Can you work these out from the drawing? Everything is in mm from the part's minimum corner. A direction names the side the tool comes from. Round coordinates to 2 decimals unless told otherwise and drop trailing zeros. Loops run counter-clockwise (first coordinate to the right, second up) from the corner with the lowest first, then second, coordinate; pieces in that order, holes last. Notation, with made-up numbers: (-3, 16) - (38, 16) arc R24 cw to (38, 31) - close; hole circle Ø4 at (56.5, 42.25). An arc over 180 degrees is marked (long way). Return JSON: item names as keys, results as strings. Group by question number.
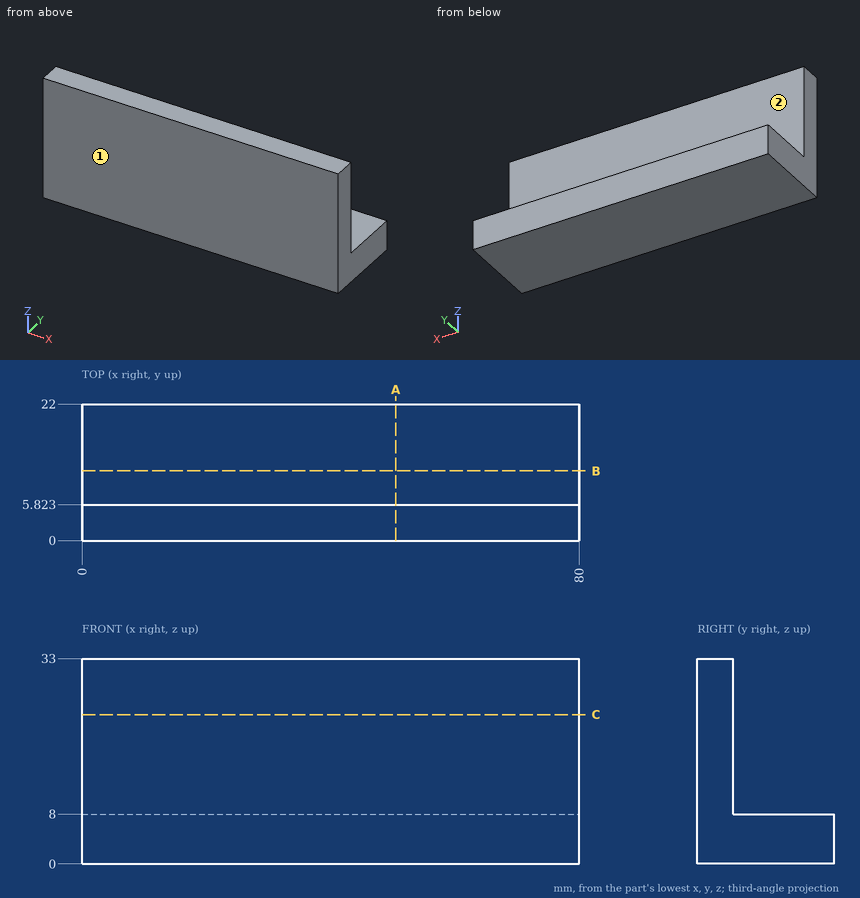
Q1. Imagine slicing it at C-C, the plane z = 24. List the corners of the cut face in (x, y) for me, and give its area (3 significant figures).
Q2. Imagine slicing it at B-B, the plane y = 11.25. List the corners of the cut face in (x, z) for me, and give its area (3 significant figures).
Q3. Imagine slicing it at A-A, the plane x = 50.5. List the corners of the cut face in (y, z) for me, and give its area (3 significant figures).
Q4. Will these pins go through, and if not, where does the flat tip stop? pin 1 Ø4 at (x, y) = (16, 6.5) entering from +Z; pin 2 Ø1.5 at (x, y) = (35, 16) entering from +Z; pin 3 Ø5 at (x, z) = (13, 20.5) entering from +Y.
Q5. Please list where these lines run through material, in increasing order: line 1 (Z direction, x = 32, y = 14.5); line 2 (Y direction, x = 59.5, z = 26.5).
Q6. For the marked faces 1 and 2, which set-ups out of +Z, -Z, +X, -X, +Y, -Y let a thin tool reach every point of the face, with its end or its side?
Output values:
{
 "1": {"outline": "(0, 0) - (80, 0) - (80, 5.82) - (0, 5.82) - close", "area": "466 mm^2"},
 "2": {"outline": "(0, 0) - (80, 0) - (80, 8) - (0, 8) - close", "area": "640 mm^2"},
 "3": {"outline": "(0, 0) - (22, 0) - (22, 8) - (5.82, 8) - (5.82, 33) - (0, 33) - close", "area": "322 mm^2"},
 "4": {"pin 1": "stops at z = 33", "pin 2": "stops at z = 8", "pin 3": "stops at y = 5.82"},
 "5": {"line 1": "z = 0 to 8", "line 2": "y = 0 to 5.82"},
 "6": {"face 1": "+Z, -Z, +X, -X, -Y", "face 2": "+Z, +X, -X, +Y"}
}
